```python
from build123d import *

# Parameters (mm, degrees)
SKETCH1_W                 = 94
SKETCH1_H                 = 136
BOSS_EXTRUDE1_DEPTH       = 1.5
FILLET1_R                 = 5
SKETCH_PATTERN1_OUTLINE_R = 1.9304
SKETCH_PATTERN1_DEPTH     = 1.5
SKETCH4_R                 = 1.8985
CUT_EXTRUDE1_DEPTH        = 137.364401513


# Read off the part's stored shape, not the designer's step: Sketch-Pattern1
with BuildPart() as part:
    # Sketch1 → Boss-Extrude1 (new body)
    with BuildSketch(Plane.XY):
        with Locations((0, 60)):
            Rectangle(SKETCH1_W, SKETCH1_H)
    extrude(amount=BOSS_EXTRUDE1_DEPTH)

    # Fillet1
    fillet1_edges = [part.edges().sort_by_distance(p)[0] for p in [
        (47, -8, 0.75),
        (-47, -8, 0.75),
        (-47, 128, 0.75),
        (47, 128, 0.75),
    ]]
    fillet(fillet1_edges, radius=FILLET1_R)

    # Sketch3 → #24 (0.152) Diameter Hole1 (revolve, cut)
    with BuildSketch(Plane(origin=(43, 0, 1.5), x_dir=(0, -1, 0), z_dir=(1, 0, 0))):
        Polygon((0, 0), (0, 13.859901339), (1.9304, 12.7), (1.9304, 0), align=None)
    revolve(axis=Axis((43, 0, 7.85), (0, 0, -1)), mode=Mode.SUBTRACT)

    # Sketch-Pattern1 outline → Sketch-Pattern1 (cut)
    with BuildSketch(Plane.XY):
        with Locations((0, -4)):
            Circle(SKETCH_PATTERN1_OUTLINE_R)
        with Locations((0, 124)):
            Circle(SKETCH_PATTERN1_OUTLINE_R)
        with Locations((43, 120)):
            Circle(SKETCH_PATTERN1_OUTLINE_R)
        with Locations((43, 60)):
            Circle(SKETCH_PATTERN1_OUTLINE_R)
        with Locations((-43, 120)):
            Circle(SKETCH_PATTERN1_OUTLINE_R)
        with Locations((-43, 60)):
            Circle(SKETCH_PATTERN1_OUTLINE_R)
        with Locations((-43, 0)):
            Circle(SKETCH_PATTERN1_OUTLINE_R)
    extrude(amount=SKETCH_PATTERN1_DEPTH, mode=Mode.SUBTRACT)

    # Sketch4 → Cut-Extrude1 (cut, through all)
    with BuildSketch(Plane(origin=(0, 0, 0), x_dir=(-1, 0, 0), z_dir=(0, 0, -1))):
        with Locations((20.500102944, 76.500016768)):
            Circle(SKETCH4_R)
        with Locations((-20.500312859, 76.499889767)):
            Circle(SKETCH4_R)
    extrude(amount=-CUT_EXTRUDE1_DEPTH, mode=Mode.SUBTRACT)


solid = part.part
```
Geometry: final body of the model. Coordinates: model frame, mm. Coordinates: 2 decimals unless noted, no trailing zeros. Loops run counter-clockwise (first coordinate to the right, second up) from the corner with the lowest first, then second, coordinate; pieces in that order, holes last. Notation, with made-up numbers: (30, 79) -> (76, 79) arc R13 ccw to (76, 89) -> close; hole circle Ø5 at (55.25, 16.25). An arc over 180 degrees is marked (long way). Use a Markdown table: item, result. Add a question column.
(1) Pin query (flat end, axial travel): pin 1 Ø8 at (x, y) = (2.5, 20.5) entering from -Z. Return the tip coordinate at first contact, or that it passes through.
(2) Section query A-A, the plane y = 0. Return loops of the section in (x, z).
(3) Section query B-B, the plane x = 20.5. Return loops of the section in (y, z), plus the area to 3 significant figures.
(4) Line query: line 1 along X through (y, z) = (120, 0.6); line 2 along Y through (x, z) = (0, 0.6); line 3 along Y through (x, z) = (-43, 0.65). Output: solid intervals per line, ascending.
(5) Mould query, pull axis Y, two halves, no side actions, for faces 1 (the cylindrical face through (45, -7, 1)), 2 (the cylindrical face through (-0.251, 125.914, 0.74)), 3 (the cylindrical face through (-46, 126, 1)). Classes: pulls with the +Y half, pulls with the -Y half, needs draft (parallel to the pull), parting line crosses it, or undercut.
Answer:
| question | item | result |
|---|---|---|
| 1 | pin 1 | stops at z = 0 |
| 2 | outline | (-47, 0) -> (-44.93, 0) -> (-44.93, 1.5) -> (-47, 1.5) -> close; (-41.07, 0) -> (41.07, 0) -> (41.07, 1.5) -> (-41.07, 1.5) -> close; (44.93, 0) -> (47, 0) -> (47, 1.5) -> (44.93, 1.5) -> close |
| 3 | outline | (-8, 0) -> (74.6, 0) -> (74.6, 1.5) -> (-8, 1.5) -> close; (78.4, 0) -> (128, 0) -> (128, 1.5) -> (78.4, 1.5) -> close |
| 3 | area | 198 mm^2 |
| 4 | line 1 | x = -47 to -44.93, -41.07 to 41.07, 44.93 to 47 |
| 4 | line 2 | y = -8 to -5.93, -2.07 to 122.07, 125.93 to 128 |
| 4 | line 3 | y = -7.9 to -1.93, 1.93 to 58.07, 61.93 to 118.07, 121.93 to 127.9 |
| 5 | face 1 | pulls with the -Y half |
| 5 | face 2 | undercut |
| 5 | face 3 | pulls with the +Y half |
